```python
from build123d import *

# Parameters (mm, degrees)
BOSS_EXTRUDE3_START       = 601
BOSS_EXTRUDE3_OUTLINE_R   = 45
BOSS_EXTRUDE3_OUTLINE_R_2 = 35
BOSS_EXTRUDE3_DEPTH       = 100
SKETCH3_R                 = 40
SKETCH3_R_2               = 35
BOSS_EXTRUDE4_DEPTH       = 20
BOSS_EXTRUDE5_START       = 20
SKETCH4_R                 = 40
SKETCH4_R_2               = 35
BOSS_EXTRUDE5_DEPTH       = 20


# Read off the part's stored shape, not the designer's step: Boss-Extrude3
with BuildPart() as part:
    # Boss-Extrude3 outline → Boss-Extrude3 (new body)
    with BuildSketch(Plane(origin=(0, 0, 0), x_dir=(1, 0, 0), z_dir=(0, 1, 0)).offset(BOSS_EXTRUDE3_START)):
        Circle(BOSS_EXTRUDE3_OUTLINE_R)
        Circle(BOSS_EXTRUDE3_OUTLINE_R_2, mode=Mode.SUBTRACT)
    extrude(amount=BOSS_EXTRUDE3_DEPTH)

    # Sketch3 → Boss-Extrude4 (add)
    with BuildSketch(Plane(origin=(0, 701, 0), x_dir=(1, 0, 0), z_dir=(0, 1, 0))):
        with Locations(Location((0, 0, 0), (0, 0, 180))):
            Circle(SKETCH3_R)
        with Locations(Location((0, 0, 0), (0, 0, 270))):
            Circle(SKETCH3_R_2, mode=Mode.SUBTRACT)
    extrude(amount=BOSS_EXTRUDE4_DEPTH)

    # Sketch4 → Boss-Extrude5 (add)
    with BuildSketch(Plane.XZ.offset(-601).offset(BOSS_EXTRUDE5_START)):
        with Locations(Location((0, 0, 0), (0, 0, 180))):
            Circle(SKETCH4_R)
        with Locations(Location((0, 0, 0), (0, 0, 180))):
            Circle(SKETCH4_R_2, mode=Mode.SUBTRACT)
    extrude(amount=-BOSS_EXTRUDE5_DEPTH)


solid = part.part
```
Design review of the part built by this model. Coordinates are the model's own, in mm. A direction names the side the tool comes from. Round coordinates to 2 decimals unless told otherwise and drop trailing zeros. Order: outer loops, then holes, each group sorted by start corner. A loop starts at its lowest first (then second) coordinate and runs counter-clockwise, first axis right, second up. Notation, with made-up numbers: (22.5, 49) - (26.5, 49) arc R14 cw to (26.5, 71) - close; hole circle Ø2 at (-19, 63.25). An arc over 180 degrees is marked (long way). Return JSON: item names as keys, results as strings.
Q1. Consider section B-B on x = 0. Write out the cut boundary in (y, z).
Computed values:
{"outline": "(581, -40) - (601, -40) - (601, -45) - (701, -45) - (701, -40) - (721, -40) - (721, -35) - (581, -35) - close; (581, 35) - (721, 35) - (721, 40) - (701, 40) - (701, 45) - (601, 45) - (601, 40) - (581, 40) - close"}
Q2. Wall thickness on L1, parallel to Z at x = 0, y = 590; L2, parallel to Z at x = 0, y = 683; L3, parallel to Y at x = 32.5, z = -29: over which ranges is each line inside the solid? List them lowest first. Write a range as [from, to].
Computed values:
{"L1": "z = [-40, -35], [35, 40]", "L2": "z = [-45, -35], [35, 45]", "L3": "y = [601, 701]"}
Q3. Consider section A-A on z = 0. Write out the cut boundary in (x, y).
Computed values:
{"outline": "(-45, 601) - (-40, 601) - (-40, 581) - (-35, 581) - (-35, 721) - (-40, 721) - (-40, 701) - (-45, 701) - close; (35, 581) - (40, 581) - (40, 601) - (45, 601) - (45, 701) - (40, 701) - (40, 721) - (35, 721) - close"}
Q4. For pin 1 Ø2 at (y, z) = (622.5, 29) entering from +X; pin 2 Ø12 at (x, z) = (-34, 27.5) entering from -Y; pin 3 Ø5 at (y, z) = (653.5, -35.5) entering from -X; pin 4 Ø1.5 at (x, y) = (-33, 689) entering from +Z, all flat-tipped, find the tip position at first contact; note any pin that passes through.
Computed values:
{"pin 1": "stops at x = 35.23", "pin 2": "stops at y = 581", "pin 3": "stops at x = -30.59", "pin 4": "stops at z = 31.38"}
Q5. Consider section C-C on y = 622.5. Write out the cut boundary in (x, z), plus the area to 3 significant figures.
Computed values:
{"outline": "circle Ø90 at (0, 0); hole circle Ø70 at (0, 0)", "area": "2,510 mm2"}
Q6. Consider section D-D on x = 38. Write out the cut boundary in (y, z).
Computed values:
{"outline": "(581, -12.49) - (601, -12.49) - (601, -24.1) - (701, -24.1) - (701, -12.49) - (721, -12.49) - (721, 12.49) - (701, 12.49) - (701, 24.1) - (601, 24.1) - (601, 12.49) - (581, 12.49) - close"}
Q7. Machinability: for faces 1 (the flat face through (-30.2, 601, 26.5)), 2 (the cylindrical face through (39.96, 710.86, 1.76)), 3 (the flat face through (0.2, 721, -35.4)), which of the approach directions +Z, -Z, +X, -X, +Y, -Y give a long, thin tool a straight path to every point of the face, cutting with its end or side? Answer none if there is none.
Computed values:
{"face 1": "-Y", "face 2": "+Y", "face 3": "+Z, -Z, +X, -X, +Y"}
